```python
from build123d import *

# Parameters (mm, degrees)
F0_W     = 160
F0_H     = 5
F1_DEPTH = 25
F0_H_2   = 10
F2_DEPTH = 5
F3_DEPTH = 25
F4_R     = 2
F5_DEPTH = 5
F6_D     = 8.5
F6_DEPTH = 2
F6_TIP   = 2.5536576309
F7_R     = 15
F8_R     = 1


with BuildPart() as f1:
    # F0 (on Top) → F1 (new body)
    with BuildSketch(Plane.XY):
        with Locations((80, 2.5)):
            Rectangle(F0_W, F0_H)
        with Locations((80, 7.5)):
            Rectangle(F0_W, F0_H)
    extrude(amount=F1_DEPTH)

    # F0 (on Top) → F2 (join)
    with BuildSketch(Plane.XY):
        with Locations((80, 15)):
            Rectangle(F0_W, F0_H_2)
    extrude(amount=F2_DEPTH)

    # F0 (on Top) → F3 (join)
    with BuildSketch(Plane.XY):
        with Locations((80, 2.5)):
            Rectangle(F0_W, F0_H)
    extrude(amount=-F3_DEPTH)

    # F4 (on face) → F5 (cut, through all)
    with BuildSketch(Plane.XZ):
        with Locations((12.5, -12.5)):
            Circle(F4_R)
        with Locations((147.5, -12.5)):
            Circle(F4_R)
    extrude(amount=-F5_DEPTH, mode=Mode.SUBTRACT)

    # F6
    with Locations(Plane.XZ):
        with Locations((12.5, -12.5), (147.5, -12.5)):
            Hole(F6_D / 2, depth=F6_DEPTH)
            with Locations((0, 0, -(F6_DEPTH + F6_TIP / 2))):  # 118° drill point
                Cone(0, F6_D / 2, F6_TIP, mode=Mode.SUBTRACT)

    # F7
    f7_edges = [f1.edges().sort_by_distance(p)[0] for p in [
        (160, 2.5, -25),
        (0, 2.5, -25),
        (160, 5, 25),
        (0, 5, 25),
    ]]
    fillet(f7_edges, radius=F7_R)

    # F8
    f8_edges = [f1.edges().sort_by_distance(p)[0] for p in [
        (0, 10, 7.5),
        (4.393398, 10, 20.606602),
        (80, 10, 5),
        (80, 10, 25),
        (160, 10, 7.5),
        (155.606602, 10, 20.606602),
        (80, 0, 25),
        (80, 20, 5),
        (0, 0, 0),
        (4.393398, 0, 20.606602),
        (4.393398, 0, -20.606602),
        (80, 0, -25),
        (155.606602, 0, 20.606602),
        (155.606602, 0, -20.606602),
        (160, 0, 0),
        (0, 15, 5),
        (160, 15, 5),
    ]]
    fillet(f8_edges, radius=F8_R)


solid = f1.part
```
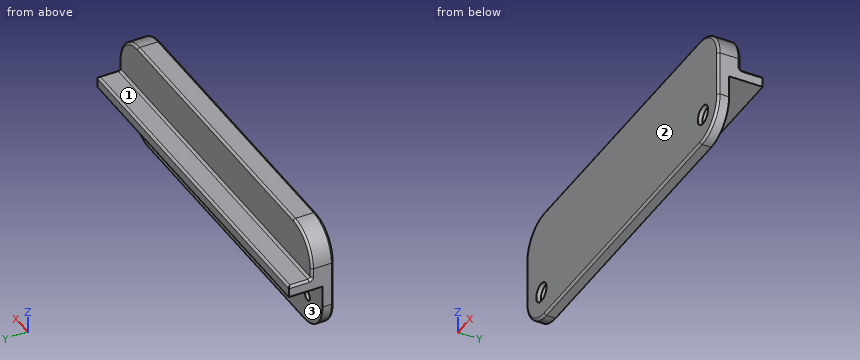
Check sheet for the modelled part. Datum: model origin and axes. Units: mm. Face numbers are marked on the shaded views. A direction names the side the tool comes from. Give positions to 0.01 mm unless a question says otherwise; leave off trailing zeros. Order: outer loops, then holes, each group sorted by start corner. A loop starts at its lowest first (then second) coordinate and runs counter-clockwise, first axis right, second up. Notation, with made-up numbers: M 0,-32.5 L 18,-32.5 A24 cw 18,-7.5 Z; hole C 57.25,82 d1. An arc over 180 degrees is marked long. Answer in a Markdown table with one row per item. Add a question column.
Q1. Sectioned sample at C-C, the plane z = -12.5. Count the separate pieces of the cut face and the enclosed holes in it, and give its area (3 significant figures).
Q2. Access from +Z, -Z, +X, -X, +Y, -Y to the whole of each face (thin tool, end or side, straight path). Record for the marked faces 1, 2 and 3.
Q3. Sectioned sample at B-B, the plane x = 30.5. Record the boundary of the cut face in (y, z), and give its area (3 significant figures).
Q4. Gauge pin test, flat ends, axial feed: pin 1 Ø4.5 at (x, z) = (147.5, -12.5) entering from -Y; pin 2 Ø12 at (y, z) = (8, 17) entering from +X; pin 3 Ø4 at (x, y) = (25.5, 9.5) entering from -Z. Record the tip position at first contact, or that the pin passes through.
Q5. Thickness scan on L1, parallel to X at y = 0.8, z = -12.5; L2, parallel to Y at x = 101, z = 8; L3, parallel to X at y = 0.65, z = -12.5. Record the ranges inside material, lowest first.
Q6. Sectioned sample at A-A, the plane z = 8. Record the boundary of the cut face in (x, y), and give its area (3 significant figures).
Verdict:
| question | item | result |
|---|---|---|
| 1 | separate pieces | 3 |
| 1 | enclosed holes | 0 |
| 1 | area | 733 mm² |
| 2 | face 1 | +Z, +X, -X, +Y |
| 2 | face 2 | +Z, -Z, +X, -X, -Y |
| 2 | face 3 | -Z, +X, -X, +Y |
| 3 | outline | M 0,-24 A1 ccw 1,-25 L 5,-25 L 5,0 L 20,0 L 20,4 A1 ccw 19,5 L 11,5 A1 cw 10,6 L 10,24 A1 ccw 9,25 L 1,25 A1 ccw 0,24 Z |
| 3 | area | 424 mm² |
| 4 | pin 1 | y = 3.2 |
| 4 | pin 2 | x = 159.97 |
| 4 | pin 3 | z = 0 |
| 5 | L1 | 0.23 to 8.25, 16.75 to 143.25, 151.75 to 159.77 |
| 5 | L2 | 0 to 10 |
| 5 | L3 | 0.27 to 8.25, 16.75 to 143.25, 151.75 to 159.73 |
| 6 | outline | M 0,1 A1 ccw 1,0 L 159,0 A1 ccw 160,1 L 160,9 A1 ccw 159,10 L 1,10 A1 ccw 0,9 Z |
| 6 | area | 1,600 mm² |
